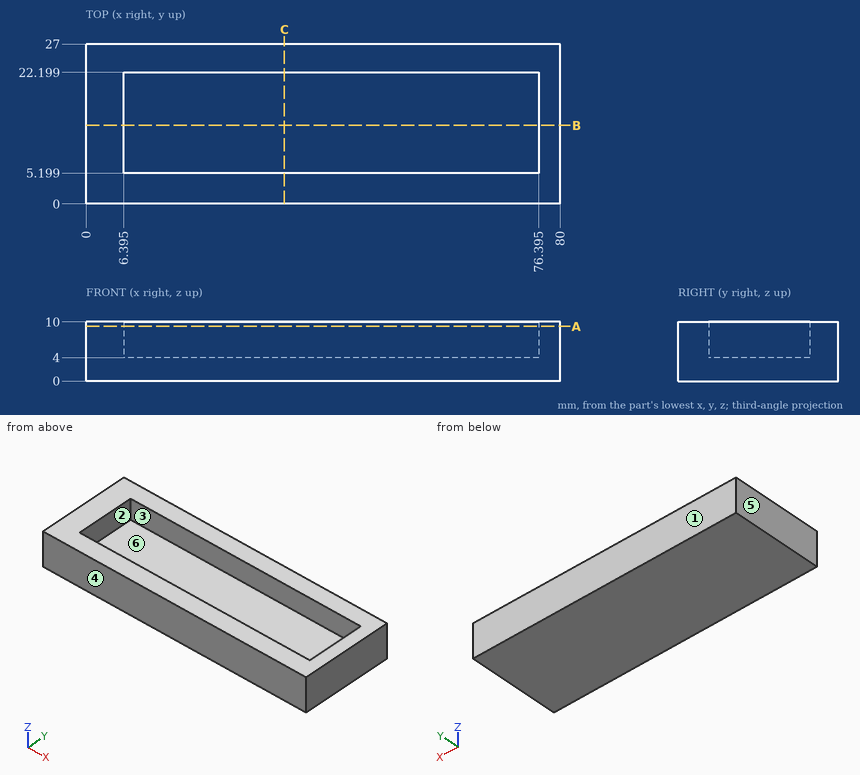
Design review of the part shown in the three views and the two pictorial views. Dimensions are in mm from the part's minimum x, y and z. A direction names the side the tool comes from. Round coordinates to 2 decimals unless told otherwise and drop trailing zeros. Loops run counter-clockwise (first coordinate to the right, second up) from the corner with the lowest first, then second, coordinate; pieces in that order, holes last.
(1) We need section C-C (x = 33.5). Give the boundary of the cut face in (y, z).
Returned:
outline: (0, 0) - (27, 0) - (27, 10) - (22.2, 10) - (22.2, 4) - (5.2, 4) - (5.2, 10) - (0, 10) - close
(2) We need section A-A (z = 9.25). Give the boundary of the cut face in (x, y) (1 decimal), plus the area to 3 significant figures.
Returned:
outline: (0, 0) - (80, 0) - (80, 27) - (0, 27) - close; hole (6.4, 5.2) - (76.4, 5.2) - (76.4, 22.2) - (6.4, 22.2) - close
area: 970 mm2
(3) Tool access review of the marked faces 1 and 2: name each direction out of +Z, -Z, +X, -X, +Y, -Y from which nothing blocks a thin tool from reaching the whole face with its end or side.
Returned:
face 1: +Z, -Z, +X, -X, +Y
face 2: +Z
(4) Mouldability with a two-part tool opening along Y and no side actions: class the marked faces 3, 4, 5 and 6 as released by +Y, released by -Y, zero draft, split by the parting line, or undercut.
Returned:
face 3: undercut
face 4: released by -Y
face 5: zero draft
face 6: undercut
(5) We need section B-B (y = 13.25). Give the boundary of the cut face in (x, z) (1 decimal).
Returned:
outline: (0, 0) - (80, 0) - (80, 10) - (76.4, 10) - (76.4, 4) - (6.4, 4) - (6.4, 10) - (0, 10) - close
(6) Wall thickness on line 1 along Y through (x, z) = (49.5, 5.25); line 2 along X through (y, z) = (18.5, 7.25) (1 decimal); line 3 along Z through (x, y) = (48, 13.5): over which ranges is each line inside the solid? List them lowest first.
Returned:
line 1: y = 0 to 5.2, 22.2 to 27
line 2: x = 0 to 6.4, 76.4 to 80
line 3: z = 0 to 4
(7) Clearance check with flat-ended pins moving along their axes: P1, Ø2, axis at x = 43, z = 4, coming from the -Y side; P2, Ø12, axis at x = 21.5, y = 15.5, coming from the +Z side. State where each tip first meets the part, or that it passes through.
Returned:
P1: stops at y = 0
P2: stops at z = 4
